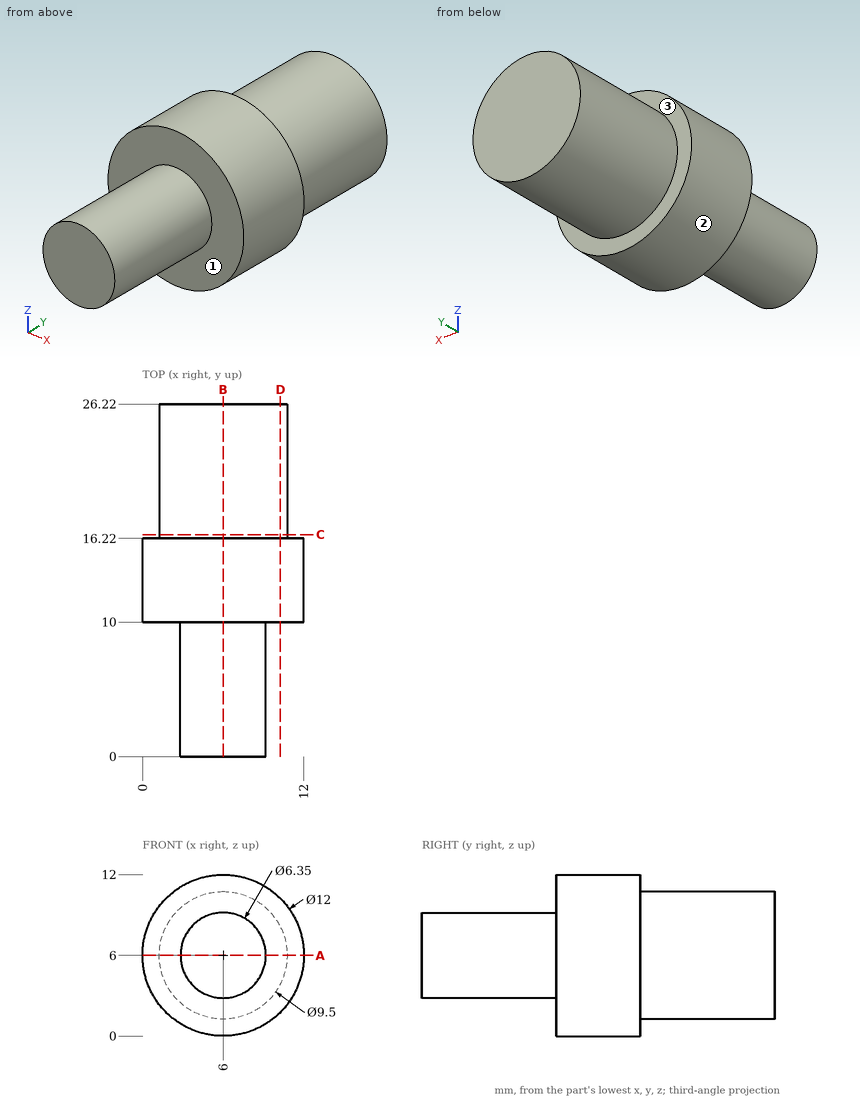
The figure shows three views and two pictorial views of one solid part (mm, origin at its lowest corner). Answer the questions. A direction names the side the tool comes from. Coordinates: 2 decimals unless noted, no trailing zeros. Loops run counter-clockwise (first coordinate to the right, second up) from the corner with the lowest first, then second, coordinate; pieces in that order, holes last.
(1) The part is cut by section D-D (x = 10.25). Determine the outline of the cut face in (y, z), and give its area (3 significant figures).
Solution:
outline: (10, 1.76) - (16.22, 1.76) - (16.22, 3.88) - (26.22, 3.88) - (26.22, 8.12) - (16.22, 8.12) - (16.22, 10.24) - (10, 10.24) - close
area: 95.1 mm2
(2) A tool of negligible diameter and unlimited length cuts with its end or side. For the marked faces 1, 2 and 3, from which of +Z, -Z, +X, -X, +Y, -Y can it reach the whole face along a straight path? Write none if from no direction.
Solution:
face 1: -Y
face 2: +Y, -Y
face 3: +Y
(3) The part is cut by section B-B (x = 6). Determine the outline of the cut face in (y, z) (3 decimals).
Solution:
outline: (0, 2.825) - (10, 2.825) - (10, 0) - (16.22, 0) - (16.22, 1.25) - (26.22, 1.25) - (26.22, 10.75) - (16.22, 10.75) - (16.22, 12) - (10, 12) - (10, 9.175) - (0, 9.175) - close
(4) Flat-ended cylindrical pins translate along their axes: pin 1 Ø3 at (x, y) = (6, 23) entering from -Z; pin 2 Ø2 at (y, z) = (14.5, 2) entering from +X; pin 3 Ø2 at (x, z) = (10.5, 10) entering from -Y. Find the tip coordinate at first contact, or state that the pin passes through.
Solution:
pin 1: stops at z = 1.25
pin 2: stops at x = 11.2
pin 3: stops at y = 10
(5) The part is cut by section A-A (z = 6). Determine the outline of the cut face in (x, y) (3 decimals), and give its area (3 significant figures).
Solution:
outline: (0, 10) - (2.825, 10) - (2.825, 0) - (9.175, 0) - (9.175, 10) - (12, 10) - (12, 16.22) - (10.75, 16.22) - (10.75, 26.22) - (1.25, 26.22) - (1.25, 16.22) - (0, 16.22) - close
area: 233 mm2
(6) The part is cut by section C-C (y = 16.5). Determine the outline of the cut face in (x, z).
Solution:
outline: circle Ø9.5 at (6, 6)
(7) Consider line 1 along Y through (x, z) = (10.75, 4.5); line 2 along Y through (x, z) = (9, 7.25); line 3 along X through (y, z) = (1, 6) (3 decimals). Determine where each line is inside the solid, lowest interval first.
Solution:
line 1: y = 10 to 16.22
line 2: y = 10 to 26.22
line 3: x = 2.825 to 9.175
